The model under review builds one solid part; all positions refer to its coordinate system, in mm. Face numbers are marked on the shaded views. A direction names the side the tool comes from. Coordinates: 2 decimals unless noted, no trailing zeros. Loops run counter-clockwise (first coordinate to the right, second up) from the corner with the lowest first, then second, coordinate; pieces in that order, holes last. Notation, with made-up numbers: (-28, 39) - (-3, 39) arc R19 ccw to (-3, 73) - close; hole circle Ø2 at (78.25, -39). An arc over 180 degrees is marked (long way). Answer in a Markdown table with one row per item. Add a question column.
(1) We need section B-B on y = 101. Write out the cut boundary in (x, z), plus the area to 3 significant figures.
(2) Machinability: for the marked faces 5 and 6, which of the approach directions +Z, -Z, +X, -X, +Y, -Y give a long, thin tool a straight path to every point of the face, cutting with its end or side? Answer none if there is none.
(3) We need section C-C on x = -405. Write out the cut boundary in (y, z).
(4) We need section A-A on z = 321.5. Write out the cut boundary in (x, y), plus the area to 3 significant figures.
(5) Mouldability with a two-part tool opening along X and no side actions: class the marked faces 1, 2, 3 and 4 as +X half, -X half, draft (parallel to the pull), parting line (faces both ways), or undercut.
(6) For line 1 along Z through (x, y) = (-69, 565.5); line 2 along Z through (x, y) = (-370, -11.5), list the stretches that pass through material, from the lowest coordinate up.
from build123d import *

# Parameters (mm, degrees)
F0_W     = 1270
F0_H     = 1270
F0_W_2   = 1016
F0_H_2   = 1016
F1_DEPTH = 635
F2_R     = 101.6
F3_SIZE  = 152.4


with BuildPart() as f1:
    # F0 (on Front) → F1 (new body, symmetric)
    with BuildSketch(Plane.XZ):
        Rectangle(F0_W, F0_H)
        Rectangle(F0_W_2, F0_H_2, mode=Mode.SUBTRACT)
    extrude(amount=F1_DEPTH, both=True)

    # F2
    f2_edges = [f1.edges().sort_by_distance(p)[0] for p in [
        (635, 0, 635),
    ]]
    fillet(f2_edges, radius=F2_R)

    # F3
    f3_edges = [f1.edges().sort_by_distance(p)[0] for p in [
        (-508, 0, -508),
    ]]
    chamfer(f3_edges, length=F3_SIZE)


solid = f1.part
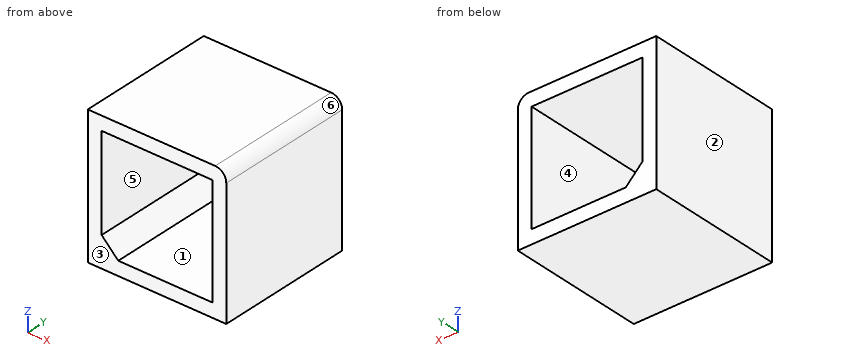
Outcome:
| question | item | result |
|---|---|---|
| 1 | outline | (-635, -635) - (635, -635) - (635, 533.4) arc R101.6 ccw to (533.4, 635) - (-635, 635) - close; hole (-508, -355.6) - (-355.6, -508) - (508, -508) - (508, 508) - (-508, 508) - close |
| 1 | area | 590,000 mm² |
| 2 | face 5 | +Y, -Y |
| 2 | face 6 | +Z, +X, +Y, -Y |
| 3 | outline | (-635, -635) - (635, -635) - (635, -458.6) - (-635, -458.6) - close; (-635, 508) - (635, 508) - (635, 635) - (-635, 635) - close |
| 4 | outline | (-635, -635) - (-508, -635) - (-508, 635) - (-635, 635) - close; (508, -635) - (635, -635) - (635, 635) - (508, 635) - close |
| 4 | area | 323,000 mm² |
| 5 | face 1 | undercut |
| 5 | face 2 | -X half |
| 5 | face 3 | draft |
| 5 | face 4 | undercut |
| 6 | line 1 | -635 to -508, 508 to 635 |
| 6 | line 2 | -635 to -493.6, 508 to 635 |
